Build history of the part. All positions in model axes, mm. Face numbers are marked on the shaded views. A direction names the side the tool comes from. Round coordinates to 2 decimals unless told otherwise and drop trailing zeros. Loops run counter-clockwise (first coordinate to the right, second up) from the corner with the lowest first, then second, coordinate; pieces in that order, holes last. Notation, with made-up numbers: (89.5, 14) -> (141.5, 14) arc R34 cw to (141.5, 53) -> close; hole circle Ø10 at (-26, 8.5). An arc over 180 degrees is marked (long way). Put each result on its own line as item: value. Start each with the question number.
Item 1: Tool access for the marked faces 4 and 5: list every direction of +Z, -Z, +X, -X, +Y, -Y with a clear straight run to the whole face (end or side of a thin tool).
Item 2: Flat gauge pins, fed straight in: pin 1 Ø0.6 at (x, y) = (-2.5, 23) entering from -Z; pin 2 Ø5.5 at (y, z) = (7.5, -15) entering from -X; pin 3 Ø6.5 at (y, z) = (18.5, -14.5) entering from -X. Where does each tip first touch, or does it go through?
Item 3: Pull direction X, two halves, no side cores. Call the marked faces 1, 2 and 3: +X half, -X half, draft (parallel to the pull), parting line (faces both ways), or undercut.
Item 4: Cut at D-D, the plane z = -22.5. List the corners of the cut face in (x, y), plus the area to 3 significant figures.
Item 5: Cut at C-C, the plane x = -23.5. List the corners of the cut face in (y, z).
Item 6: Cut at B-B, the plane y = 22. List the corners of the cut face in (x, z), plus the area to 3 significant figures.
Item 7: Cut at A-A, the plane z = -15. List the corners of the cut face in (x, y), plus the area to 3 significant figures.
Item 8: Drill centre lines: probe 1 along Y at (x, z) = (-4.25, -15); probe 2 along Y at (x, z) = (-1.15, -15); probe 3 along X at (y, z) = (4.5, -30). Where is each one in solid material? Low to high. Write a range as [from, to].
```python
from build123d import *

# Parameters (mm, degrees)
BOSS_EXTRUDE1_DEPTH = 25
CUT_EXTRUDE1_DEPTH  = 25
CUT_EXTRUDE2_DEPTH  = 25
FILLET1_R           = 1.5
SKETCH5_R           = 1.25
CUT_EXTRUDE4_DEPTH  = 25
CUT_EXTRUDE5_START  = -2.5
SKETCH5_4_R         = 3
SKETCH5_4_R_2       = 1.25
CUT_EXTRUDE5_DEPTH  = 2.5
SKETCH7_W           = 10
SKETCH7_H           = 3
CUT_EXTRUDE6_DEPTH  = 69.271516755
CHAMFER1_SIZE       = 2.5
FILLET2_R           = 1.5
CHAMFER2_SIZE       = 1.5


with BuildPart() as part:
    # Sketch1 → Boss-Extrude1 (new body)
    with BuildSketch(Plane(origin=(0, 0, 0), x_dir=(1, 0, 0), z_dir=(0, 1, 0))):
        Polygon((0, 0), (-30, 0), (-30, 5), (-5, 5), (-5, 56), (0, 56), align=None)
    extrude(amount=BOSS_EXTRUDE1_DEPTH)

    # Sketch2 → Cut-Extrude1 (cut)
    with BuildSketch(Plane(origin=(0, 0, 0), x_dir=(0, 0, -1), z_dir=(1, 0, 0))):
        Polygon((56, 25), (56, 19.253030332), (35, 21.460219273), (35, 25), align=None)
        with BuildLine():
            Line((56, 12.5), (56, 19.253030332))
            Line((56, 19.253030332), (49.283963462, 19.958914217))
            ThreePointArc((49.283963462, 19.958914217), (54.073586187, 17.518479552), (56, 12.5))
        make_face()
        with BuildLine():
            Line((56, 5.746969668), (56, 12.5))
            ThreePointArc((56, 12.5), (54.073586128, 7.481520383), (49.283963288, 5.041085765))
            Line((49.283963288, 5.041085765), (56, 5.746969668))
        make_face()
        Polygon((56, 5.746969668), (56, 0), (35, 0), (35, 3.539780727), align=None)
    extrude(amount=-CUT_EXTRUDE1_DEPTH, mode=Mode.SUBTRACT)

    # Sketch3 → Cut-Extrude2 (cut)
    with BuildSketch(Plane(origin=(0, 0, 0), x_dir=(0, 0, -1), z_dir=(1, 0, 0))):
        with BuildLine():
            Line((35, 15.5), (48.5, 15.5))
            ThreePointArc((48.5, 15.5), (51.5, 12.5), (48.5, 9.5))
            Line((48.5, 9.5), (35, 9.5))
            ThreePointArc((35, 9.5), (32, 12.5), (35, 15.5))
        make_face()
    extrude(amount=-CUT_EXTRUDE2_DEPTH, mode=Mode.SUBTRACT)

    # Fillet1
    fillet1_edges = [part.edges().sort_by_distance(p)[0] for p in [
        (-2.5, 25, -35),
        (-2.5, 21.460219273, -35),
        (-2.5, 0, -35),
        (-2.5, 3.539780727, -35),
    ]]
    fillet(fillet1_edges, radius=FILLET1_R)

    # Sketch5 → Cut-Extrude4 (cut)
    with BuildSketch(Plane(origin=(0, 0, 0), x_dir=(0, 0, -1), z_dir=(1, 0, 0))):
        with Locations((15, 17.5)):
            Circle(SKETCH5_R)
        with Locations((15, 7.5)):
            Circle(SKETCH5_R)
    extrude(amount=-CUT_EXTRUDE4_DEPTH, mode=Mode.SUBTRACT)

    # Sketch5_4 → Cut-Extrude5 (cut)
    # profile 1 of 2: a face of its own
    with BuildSketch(Plane(origin=(0, 0, 0), x_dir=(0, 0, -1), z_dir=(1, 0, 0)).offset(CUT_EXTRUDE5_START)):
        with Locations((15, 17.5)):
            Circle(SKETCH5_4_R)
        with Locations((15, 17.5)):
            Circle(SKETCH5_4_R_2, mode=Mode.SUBTRACT)
    # profile 2 of 2: a face of its own
    with BuildSketch(Plane(origin=(0, 0, 0), x_dir=(0, 0, -1), z_dir=(1, 0, 0)).offset(CUT_EXTRUDE5_START)):
        with Locations((15, 7.5)):
            Circle(SKETCH5_4_R)
        with Locations((15, 7.5)):
            Circle(SKETCH5_4_R_2, mode=Mode.SUBTRACT)
    extrude(amount=-CUT_EXTRUDE5_DEPTH, mode=Mode.SUBTRACT)

    # Sketch7 → Cut-Extrude6 (cut, through all)
    with BuildSketch(Plane(origin=(0, 25, 0), x_dir=(1, 0, 0), z_dir=(0, 1, 0))):
        with Locations((-15, 1.5)):
            Rectangle(SKETCH7_W, SKETCH7_H)
    extrude(amount=-CUT_EXTRUDE6_DEPTH, mode=Mode.SUBTRACT)

    # Chamfer1
    chamfer1_edges = [part.edges().sort_by_distance(p)[0] for p in [
        (0, 12.5, 0),
        (-30, 12.5, 0),
    ]]
    chamfer(chamfer1_edges, length=CHAMFER1_SIZE)

    # Fillet2
    fillet2_edges = [part.edges().sort_by_distance(p)[0] for p in [
        (-5, 12.5, -5),
        (-30, 12.5, -5),
    ]]
    fillet(fillet2_edges, radius=FILLET2_R)

    # Chamfer2
    chamfer2_edges = [part.edges().sort_by_distance(p)[0] for p in [
        (-5, 9.5, -41.75),
        (-5, 12.5, -51.5),
        (-5, 15.5, -41.75),
        (-5, 12.5, -32),
    ]]
    chamfer(chamfer2_edges, length=CHAMFER2_SIZE)


solid = part.part
```
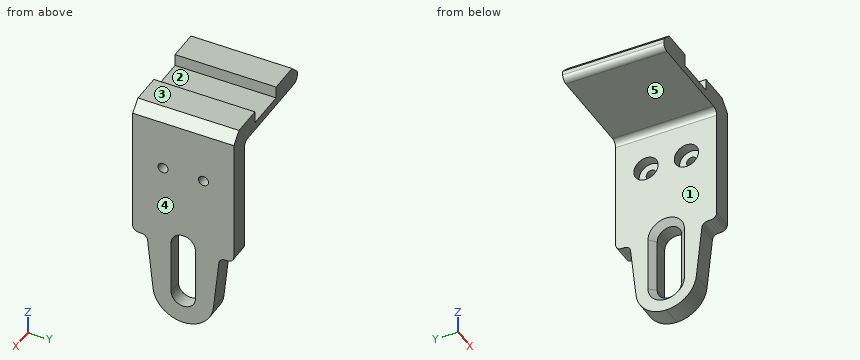
Reply:
1. face 4: +Z, -Z, +X, +Y, -Y
1. face 5: -Z, -X, +Y, -Y
2. pin 1: stops at z = -35
2. pin 2: stops at x = -2.5
2. pin 3: stops at x = -5
3. face 1: -X half
3. face 2: undercut
3. face 3: draft
4. outline: (-5, 0) -> (0, 0) -> (0, 25) -> (-5, 25) -> close
4. area: 125 mm^2
5. outline: (0, -5) -> (25, -5) -> (25, 0) -> (0, 0) -> close
6. outline: (-30, -3.5) arc R1.5 ccw to (-28.5, -5) -> (-6.5, -5) arc R1.5 cw to (-5, -6.5) -> (-5, -35.24) -> (0, -35.24) -> (0, -2.5) -> (-2.5, 0) -> (-10, 0) -> (-10, -3) -> (-20, -3) -> (-20, 0) -> (-27.5, 0) -> (-30, -2.5) -> close
6. area: 265 mm^2
7. outline: (-5, 0) -> (0, 0) -> (0, 6.25) -> (-2.5, 6.25) -> (-2.5, 4.5) -> (-5, 4.5) -> close; (-5, 10.5) -> (-2.5, 10.5) -> (-2.5, 8.75) -> (0, 8.75) -> (0, 16.25) -> (-2.5, 16.25) -> (-2.5, 14.5) -> (-5, 14.5) -> close; (-5, 20.5) -> (-2.5, 20.5) -> (-2.5, 18.75) -> (0, 18.75) -> (0, 25) -> (-5, 25) -> close
7. area: 82.5 mm^2
8. probe 1: y = [0, 4.5], [10.5, 14.5], [20.5, 25]
8. probe 2: y = [0, 6.25], [8.75, 16.25], [18.75, 25]
8. probe 3: x = [-5, 0]
